from build123d import *

# Parameters (mm, degrees)
F1_W      = 34.5
F1_H      = 32
F2_DEPTH  = 3
F3_R      = 3
F4_W      = 28.5
F4_H      = 26
F5_DEPTH  = 7
F6_W      = 6
F6_H      = 6
F6_W_2    = 3
F6_H_2    = 3
F7_DEPTH  = 3
F8_W      = 10.5
F8_H      = 1
F9_DEPTH  = 3
F10_W     = 1
F10_H     = 4
F11_DEPTH = 34.5
F13_DEPTH = 7
F14_R     = 1
F15_R     = 0.6


with BuildPart() as f2:
    # F1 (on Top) → F2 (new body)
    with BuildSketch(Plane.XY):
        Rectangle(F1_W, F1_H)
    extrude(amount=F2_DEPTH)

    # F3
    f3_edges = [f2.edges().sort_by_distance(p)[0] for p in [
        (17.25, -16, 1.5),
        (-17.25, -16, 1.5),
        (17.25, 16, 1.5),
        (-17.25, 16, 1.5),
    ]]
    fillet(f3_edges, radius=F3_R)

    # F4 (on face) → F5 (join)
    with BuildSketch(Plane.XY.offset(3)):
        with BuildLine():
            ThreePointArc((14.25, -16), (16.3713203436, -15.1213203436), (17.25, -13))
            Line((17.25, -13), (17.25, 13))
            ThreePointArc((17.25, 13), (16.3713203436, 15.1213203436), (14.25, 16))
            Line((14.25, 16), (-14.25, 16))
            ThreePointArc((-14.25, 16), (-16.3713203436, 15.1213203436), (-17.25, 13))
            Line((-17.25, 13), (-17.25, -13))
            ThreePointArc((-17.25, -13), (-16.3713203436, -15.1213203436), (-14.25, -16))
            Line((-14.25, -16), (14.25, -16))
        make_face()
        Rectangle(F4_W, F4_H, mode=Mode.SUBTRACT)
    extrude(amount=F5_DEPTH)

    # F6 (on face) → F7 (join)
    with BuildSketch(Plane.XY.offset(3)):
        with Locations((-11.25, 0)):
            Rectangle(F6_W, F6_H)
        with Locations((11.25, 0)):
            Rectangle(F6_W, F6_H)
        with Locations((-12.75, 11.5)):
            Rectangle(F6_W_2, F6_H_2)
        with Locations((12.75, 11.5)):
            Rectangle(F6_W_2, F6_H_2)
        with Locations((-12.75, -11.5)):
            Rectangle(F6_W_2, F6_H_2)
        with Locations((12.75, -11.5)):
            Rectangle(F6_W_2, F6_H_2)
    extrude(amount=F7_DEPTH)

    # F8 (on face) → F9 (cut, through all)
    with BuildSketch(Plane.XZ.offset(16)):
        with Locations((-6.5, 9.5)):
            Rectangle(F8_W, F8_H)
    extrude(amount=-F9_DEPTH, mode=Mode.SUBTRACT)

    # F10 (on face) → F11 (cut, through all)
    with BuildSketch(Plane.YZ.offset(17.25)):
        with Locations((-4.5, 8)):
            Rectangle(F10_W, F10_H)
        with Locations((3.5, 8)):
            Rectangle(F10_W, F10_H)
    extrude(amount=-F11_DEPTH, mode=Mode.SUBTRACT)

    # F12 (on face) → F13 (join, through all)
    with BuildSketch(Plane(origin=(0, 3, 0), x_dir=(-1, 0, 0), z_dir=(0, 1, 0))):
        Polygon((-14.25, 10), (-14.25, 7.8), (-12.25, 7.8), align=None)
        Polygon((14.25, 10), (12.25, 7.8), (14.25, 7.8), align=None)
    extrude(amount=-F13_DEPTH)

    # F14
    f14_edges = [f2.edges().sort_by_distance(p)[0] for p in [
        (8.25, 3, 4.5),
        (8.25, -3, 4.5),
        (11.25, -10, 4.5),
        (11.25, 10, 4.5),
        (-11.25, -10, 4.5),
        (-11.25, 10, 4.5),
        (-8.25, 3, 4.5),
        (-8.25, -3, 4.5),
    ]]
    fillet(f14_edges, radius=F14_R)

    # F15
    f15_edges = [f2.edges().sort_by_distance(p)[0] for p in [
        (12.25, -0.5, 7.8),
        (-12.25, -0.5, 7.8),
    ]]
    fillet(f15_edges, radius=F15_R)


solid = f2.part
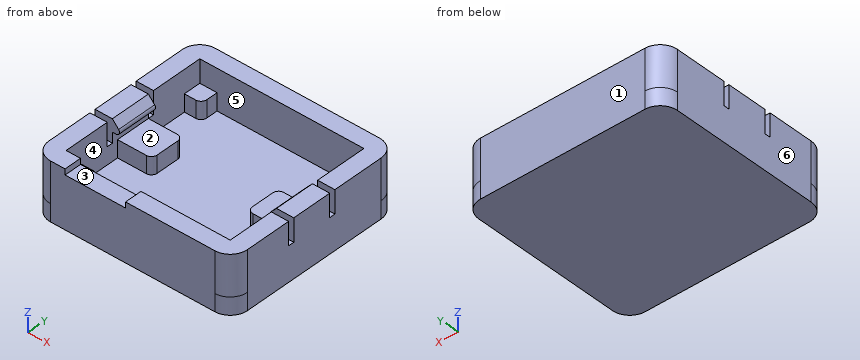
Check sheet for the modelled part. Datum: model origin and axes. Units: mm. Face numbers are marked on the shaded views. A direction names the side the tool comes from. Give positions to 0.01 mm unless a question says otherwise; leave off trailing zeros. Write each loop counter-clockwise with the first axis right and the second up, starting at its lowest first coordinate (ties: lowest second). Pieces come first, ordered by that corner, then holes. Notation, with made-up numbers: (74.25, -19) -> (100.25, -19) arc R26 ccw to (100.25, 4) -> close; hole circle Ø8 at (-32.75, 3.25). An arc over 180 degrees is marked (long way). Use one line per item in the form item = value. Start each with the question number.
1. Access from +Z, -Z, +X, -X, +Y, -Y to the whole of each face (thin tool, end or side, straight path). Record for the marked faces 4, 5 and 6.
2. Section check A-A (x = 1.5). Record the cut outline in (y, z), and give its area (3 significant figures).
3. Thickness scan on line 1 along Y through (x, z) = (-10, 4.75); line 2 along Y through (x, z) = (14, 3.75); line 3 along Y through (x, z) = (6, 9.25). Record the ranges inside material, lowest first. Write a range as from..to.
4. Section check B-B (y = 4.5). Record the cut outline in (x, z).
5. Mould release check, pull along Y, two halves, no side actions. Record for the marked faces 1, 2 and 3: pulls with the +Y half, pulls with the -Y half, needs draft (parallel to the pull), parting line crosses it, or undercut.
6. Section check C-C (y = 12.5). Record the cut outline in (x, z).
7. Go/stop test with flat-tipped pins: P1, Ø0.5, axis at x = -15, y = -4.5, coming from the +Z side; P2, Ø1.1, axis at y = -14.5, z = 9.5, coming from the -X side; P3, Ø6.5, axis at x = -10, y = -1, coming from the +Z side. Record where each tip stops, or that it passes through.
Conclusion:
q1.face_4 = none
q1.face_5 = +Z
q1.face_6 = +Z, -Z, -X, +Y, -Y
q2.outline = (-16, 0) -> (16, 0) -> (16, 10) -> (13, 10) -> (13, 3) -> (-13, 3) -> (-13, 10) -> (-16, 10) -> close
q2.area = 138 mm²
q3.line_1 = -16..-13, -3..3, 13..16
q3.line_2 = -16..-10, -3..3, 10..16
q3.line_3 = -16..-13, 13..16
q4.outline = (-17.25, 0) -> (17.25, 0) -> (17.25, 10) -> (14.25, 10) -> (14.25, 3) -> (-14.25, 3) -> (-14.25, 10) -> (-17.25, 10) -> close
q5.face_1 = pulls with the +Y half
q5.face_2 = undercut
q5.face_3 = needs draft
q6.outline = (-17.25, 0) -> (17.25, 0) -> (17.25, 10) -> (14.25, 10) -> (14.25, 6) -> (11.25, 6) -> (11.25, 3) -> (-11.25, 3) -> (-11.25, 6) -> (-14.25, 6) -> (-14.25, 10) -> (-17.25, 10) -> close
q7.P1 = 6
q7.P2 = -17.1
q7.P3 = 8.9
